Can you work these out from the model? Positions are in its coordinate system, mm. A direction names the side the tool comes from. Coordinates: 2 decimals unless noted, no trailing zeros. Loops run counter-clockwise (first coordinate to the right, second up) from the corner with the lowest first, then second, coordinate; pieces in that order, holes last.
```python
from build123d import *

# Parameters (mm, degrees)
F1_DEPTH = 25.4
F2_R     = 3.4757285613
F3_DEPTH = 25.401
F6_R     = 2.2115163873


# Not quite as in the source:
# - the program builds the solid bodies; features that only make, move or delete a surface that nothing else refers to are left out


with BuildPart() as f1:
    # F0 (on Front) → F1 (new body)
    with BuildSketch(Plane.XZ):
        Polygon((-13.319584541, 37.2763350606), (-13.319584541, 0), (-32.3739908636, 0), (-13.319584541, -18.7769141048), (-13.319584541, -51.7058856785), (13.1345912814, -51.7058856785), (13.1345912814, -18.221931532), (32.3739871383, 0), (13.1345912814, 0), (13.1345912814, 37.2763350606), (0, 51.3358972967), align=None)
    extrude(amount=F1_DEPTH)

    # F2 (on Front) → F3 (cut, through all)
    with BuildSketch(Plane.XZ):
        with Locations((0, -22.8467863053)):
            Circle(F2_R)
        with Locations((0, -30.6165441871)):
            Circle(F2_R)
        with Locations((0, -38.3863002062)):
            Circle(F2_R)
        with Locations((0, -46.5260483325)):
            Circle(F2_R)
    extrude(amount=F3_DEPTH, mode=Mode.SUBTRACT)

    # F6
    f6_edges = [f1.edges().sort_by_distance(p)[0] for p in [
        (-32.373991, -12.7, 0),
        (32.373987, -12.7, 0),
        (-13.319585, -12.7, -51.705886),
        (13.134591, -12.7, -51.705886),
        (0, -12.7, 51.335897),
    ]]
    fillet(f6_edges, radius=F6_R)


solid = f1.part
```
Item 1: Suppose I cut it at D-D, the plane x = -16. Please give me the cut outline in (y, z).
Results are:
outline: (-25.4, -16.14) - (0, -16.14) - (0, 0) - (-25.4, 0) - close
Item 2: We'd pull the mould along X, two halves only. Please class faces 1 (the face through (-0.8, -12.5, -34)), 2 (the face through (-0.03, -12.88, 50.32)), 3 (the face through (-7.386, -12.522, 43.539)): +X half, -X half, draft (parallel to the pull), parting line (faces both ways), or undercut.
Results are:
face 1: undercut
face 2: parting line
face 3: -X half
Item 3: On a 3-axis mill with a long thin cutter (end or side, diameter ignored), from which of +Z, -Z, +X, -X, +Y, -Y can I reach the whole of each face in a straight line? I mean faces 4 (the face through (-13.32, -13, 19)), 5 (the face through (-13.32, -13, -34)), 6 (the face through (13.135, -13, -34)). Say none if no direction works.
Results are:
face 4: +Z, -X, +Y, -Y
face 5: -Z, -X, +Y, -Y
face 6: -Z, +X, +Y, -Y
Item 4: Suppose I cut it at B-B, the plane z = -45. Please give me the cut outline in (x, y), plus the area to 3 significant figures.
Results are:
outline: (-13.32, -25.4) - (-3.12, -25.4) - (-3.12, 0) - (-13.32, 0) - close; (3.12, -25.4) - (13.13, -25.4) - (13.13, 0) - (3.12, 0) - close
area: 513 mm2
Item 5: I'm going to push flat-ended pins straight in: P1, Ø6, axis at y = -14, z = 5, coming from the +X side; P2, Ø5.5, axis at x = 0, z = -22.85, coming from the +Y side; P3, Ø5, axis at x = 17.5, y = -22.5, coming from the -Z side; P4, Ø2, axis at x = 18.5, y = -21.5, coming from the +Z side. Where does each tip first touch, or does it pass through?
Results are:
P1: stops at x = 13.13
P2: passes through
P3: stops at z = -16.46
P4: stops at z = 0
Item 6: Suppose I cut it at C-C, the plane y = -8.25. Please give me the cut outline in (x, z).
Results are:
outline: (-28.53, -3.79) - (-13.32, -18.78) - (-13.32, -49.49) arc R2.21 ccw to (-11.11, -51.71) - (10.92, -51.71) arc R2.21 ccw to (13.13, -49.49) - (13.13, -18.22) - (28.34, -3.82) arc R2.21 ccw to (26.82, 0) - (13.13, 0) - (13.13, 37.28) - (1.6, 49.62) arc R2.21 ccw to (-1.62, 49.63) - (-13.32, 37.28) - (-13.32, 0) - (-26.98, 0) arc R2.21 ccw to start; hole circle Ø6.95 at (0, -46.53); hole circle Ø6.95 at (0, -38.39); hole circle Ø6.95 at (0, -30.62); hole circle Ø6.95 at (0, -22.85)
Item 7: Suppose I cut it at A-A, the plane x = 0. Please give me the cut outline in (y, z).
Results are:
outline: (-25.4, -51.71) - (0, -51.71) - (0, -50) - (-25.4, -50) - close; (-25.4, -43.05) - (0, -43.05) - (0, -41.86) - (-25.4, -41.86) - close; (-25.4, -34.91) - (0, -34.91) - (0, -34.09) - (-25.4, -34.09) - close; (-25.4, -27.14) - (0, -27.14) - (0, -26.32) - (-25.4, -26.32) - close; (-25.4, -19.37) - (0, -19.37) - (0, 50.32) - (-25.4, 50.32) - close
Item 8: I need wall thicknesses on line 1 along Z through (x, y) = (0, -10.5); line 2 along X through (y, z) = (-4.25, 34); line 3 along X through (y, z) = (-17, -22). Which ranges of each line are inside material? Lowest first, please.
Results are:
line 1: z = -51.71 to -50, -43.05 to -41.86, -34.91 to -34.09, -27.14 to -26.32, -19.37 to 50.32
line 2: x = -13.32 to 13.13
line 3: x = -13.32 to -3.37, 3.37 to 13.13
